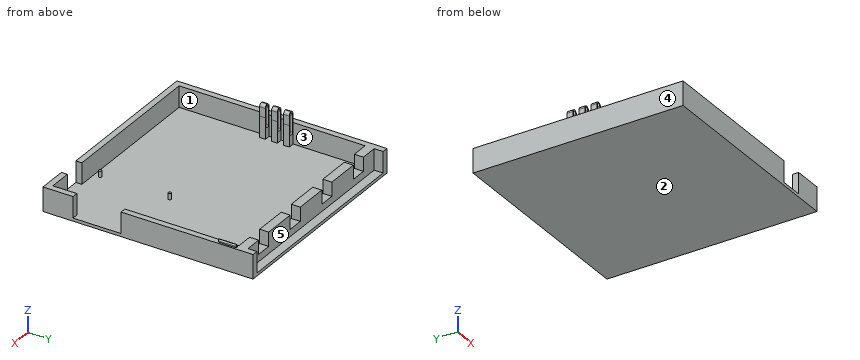
from build123d import *

# Parameters (mm, degrees)
F0_W           = 175
F0_H           = 175
F1_DEPTH       = 20
F2_W           = 165
F2_H           = 155
F3_DEPTH       = 17.5
F4_R           = 1.25
F5_DEPTH       = 5
F6_W           = 165
F6_H           = 7.5
F7_DEPTH       = 17.5
F8_W           = 13.2
F8_H           = 5.7
F9_DEPTH       = 8.5
F10_W          = 5
F10_H          = 5
F11_DEPTH      = 17.5
F11_DEPTH_BACK = 10
F11_TAPER_BACK = 1
F12_T1_DEPTH   = 16.9346144904
F12_T3_DEPTH   = 16.9346144904
F12_T5_DEPTH   = 16.9346144904
F14_DEPTH      = 25
F15_W          = 19
F15_H          = 17.6808023453
F15_W_2        = 32.2772479057
F15_H_2        = 40
F16_DEPTH      = 17.5
F17_W          = 13.2
F17_H          = 5.9
F18_DEPTH      = 8.5
F19_W          = 2
F19_H          = 15
F20_DEPTH      = 2
F21_R          = 0.99999
F22_R          = 0.5


# Not quite as in the source:
# - a fillet or chamfer that OpenCascade refuses, or shapes differently, is made with other operations: its cross-section is extruded or revolved along the edge and cut away or added
# - a fillet or chamfer is up to 0.001 mm smaller than in the source, because OpenCascade refuses the exact size


with BuildPart() as f1:
    # F0 (on Top) → F1 (new body)
    with BuildSketch(Plane.XY):
        Rectangle(F0_W, F0_H)
    extrude(amount=F1_DEPTH)

    # F2 (on face) → F3 (cut)
    with BuildSketch(Plane.XY.offset(20)):
        with Locations((0, -5)):
            Rectangle(F2_W, F2_H)
    extrude(amount=-F3_DEPTH, mode=Mode.SUBTRACT)

    # F4 (on face) → F5 (join)
    with BuildSketch(Plane.XY.offset(2.5)):
        with Locations((28.5, -77.5)):
            Circle(F4_R)
        with Locations((28.5, -19.5)):
            Circle(F4_R)
        with Locations((77.5, -77.5)):
            Circle(F4_R)
        with Locations((77.5, -19.5)):
            Circle(F4_R)
    extrude(amount=F5_DEPTH)

    # F6 (on face) → F7 (cut)
    with BuildSketch(Plane.XY.offset(20)):
        with Locations((0, 83.75)):
            Rectangle(F6_W, F6_H)
    extrude(amount=-F7_DEPTH, mode=Mode.SUBTRACT)

    # F8 (on face) → F9 (cut)
    with BuildSketch(Plane(origin=(0, 80, 0), x_dir=(-1, 0, 0), z_dir=(0, 1, 0))):
        with Locations((-61.875, 11.25)):
            Rectangle(F8_W, F8_H)
        with Locations((-20.625, 11.25)):
            Rectangle(F8_W, F8_H)
        with Locations((20.625, 11.25)):
            Rectangle(F8_W, F8_H)
        with Locations((61.875, 11.25)):
            Rectangle(F8_W, F8_H)
    extrude(amount=-F9_DEPTH, mode=Mode.SUBTRACT)

    # F10 (on face) → F11 (join, two sides)
    with BuildSketch(Plane.XY.offset(20)) as f11_sk:
        with Locations((-80, 0)):
            Rectangle(F10_W, F10_H)
        with Locations((-80, 10)):
            Rectangle(F10_W, F10_H)
        with Locations((-80, -10)):
            Rectangle(F10_W, F10_H)
    extrude(amount=-F11_DEPTH)
    extrude(f11_sk.sketch, amount=F11_DEPTH_BACK, taper=F11_TAPER_BACK)

    # F12: fillet of radius 2.5 on 6 edges, made by hand

    # F12_s2 → F12_t1 (cut)
    with BuildSketch(Plane.XZ.offset(-18.4673072452)):
        with BuildLine():
            ThreePointArc((-82.3683254308, 27.5436310161), (-81.6209793537, 29.2831261229), (-79.8687061929, 30))
            Line((-79.8687061929, 30), (-82.3254493507, 30))
            Line((-82.3254493507, 30), (-82.3683254308, 27.5436310161))
        make_face()
        with BuildLine():
            ThreePointArc((-80.1312938071, 30), (-78.3790206463, 29.2831261229), (-77.6316745692, 27.5436310161))
            Line((-77.6316745692, 27.5436310161), (-77.6745506493, 30))
            Line((-77.6745506493, 30), (-80.1312938071, 30))
        make_face()
    extrude(amount=F12_T1_DEPTH, mode=Mode.SUBTRACT)

    # F12_s4 → F12_t3 (cut)
    with BuildSketch(Plane.XZ.offset(-8.4673072452)):
        with BuildLine():
            ThreePointArc((-82.3683254308, 27.5436310161), (-81.6209793537, 29.2831261229), (-79.8687061929, 30))
            Line((-79.8687061929, 30), (-82.3254493507, 30))
            Line((-82.3254493507, 30), (-82.3683254308, 27.5436310161))
        make_face()
        with BuildLine():
            ThreePointArc((-80.1312938071, 30), (-78.3790206463, 29.2831261229), (-77.6316745692, 27.5436310161))
            Line((-77.6316745692, 27.5436310161), (-77.6745506493, 30))
            Line((-77.6745506493, 30), (-80.1312938071, 30))
        make_face()
    extrude(amount=F12_T3_DEPTH, mode=Mode.SUBTRACT)

    # F12_s6 → F12_t5 (cut)
    with BuildSketch(Plane.XZ.offset(1.5326927548)):
        with BuildLine():
            ThreePointArc((-82.3683254308, 27.5436310161), (-81.6209793537, 29.2831261229), (-79.8687061929, 30))
            Line((-79.8687061929, 30), (-82.3254493507, 30))
            Line((-82.3254493507, 30), (-82.3683254308, 27.5436310161))
        make_face()
        with BuildLine():
            ThreePointArc((-80.1312938071, 30), (-78.3790206463, 29.2831261229), (-77.6316745692, 27.5436310161))
            Line((-77.6316745692, 27.5436310161), (-77.6745506493, 30))
            Line((-77.6745506493, 30), (-80.1312938071, 30))
        make_face()
    extrude(amount=F12_T5_DEPTH, mode=Mode.SUBTRACT)

    # F13 (on face) → F14 (cut)
    with BuildSketch(Plane(origin=(0, 12.5, 0), x_dir=(-1, 0, 0), z_dir=(0, 1, 0))):
        with BuildLine():
            Line((81.5, 12.5), (81.5, 27.5))
            ThreePointArc((81.5, 27.5), (80, 29), (78.5, 27.5))
            Line((78.5, 27.5), (78.5, 12.5))
            ThreePointArc((78.5, 12.5), (80, 11), (81.5, 12.5))
        make_face()
    extrude(amount=-F14_DEPTH, mode=Mode.SUBTRACT)

    # F15 (on face) → F16 (cut)
    with BuildSketch(Plane.XY.offset(20)):
        with Locations((54, -82.5)):
            Rectangle(F15_W, F15_H)
        with Locations((82.5, -42.5)):
            Rectangle(F15_W_2, F15_H_2)
    extrude(amount=-F16_DEPTH, mode=Mode.SUBTRACT)

    # F17 (on face) → F18 (cut)
    with BuildSketch(Plane(origin=(0, 80, 0), x_dir=(-1, 0, 0), z_dir=(0, 1, 0))):
        with Locations((-61.875, 17.05)):
            Rectangle(F17_W, F17_H)
        with Locations((-20.625, 17.05)):
            Rectangle(F17_W, F17_H)
        with Locations((20.625, 17.05)):
            Rectangle(F17_W, F17_H)
        with Locations((61.875, 17.05)):
            Rectangle(F17_W, F17_H)
    extrude(amount=-F18_DEPTH, mode=Mode.SUBTRACT)

    # F19 (on face) → F20 (join)
    with BuildSketch(Plane.XY.offset(20)):
        with Locations((85, 65)):
            Rectangle(F19_W, F19_H)
    extrude(amount=F20_DEPTH)

    # F21 (radius 1 in the source; OpenCascade refuses exactly that, so slightly less here)
    f21_edges = [f1.edges().sort_by_distance(p)[0] for p in [
        (84, 65, 22),
        (86, 65, 22),
    ]]
    fillet(f21_edges, radius=F21_R)

    # F22
    f22_edges = [f1.edges().sort_by_distance(p)[0] for p in [
        (85.70711, 57.5, 21.70711),
        (85.70711, 72.5, 21.70711),
        (86, 57.5, 20.500005),
        (86, 72.5, 20.500005),
        (84, 57.5, 20.500005),
        (84.29289, 57.5, 21.70711),
        (85, 57.5, 22),
        (85, 72.5, 22),
        (84, 72.5, 20.500005),
        (84.29289, 72.5, 21.70711),
    ]]
    fillet(f22_edges, radius=F22_R)


solid = f1.part
CAD build for the part. Positions are in the model's coordinates, mm. Face numbers are marked on the shaded views. A direction names the side the tool comes from. Round coordinates to 2 decimals unless told otherwise and drop trailing zeros. Loops run counter-clockwise (first coordinate to the right, second up) from the corner with the lowest first, then second, coordinate; pieces in that order, holes last.
(1) Cut at C-C (z = 17.5). State how many separate pieces and enclosed holes the cut face has, plus the area to 3 significant figures.
(2) Cut at A-A (y = -37.5). Give the cut face in (x, z).
(3) Wall check: line 1 along X through (y, z) = (-66.5, 9.5); line 2 along Y through (x, z) = (-44, 12); line 3 along X through (y, z) = (10, 11.5). Give the ranges that are in metal, low to high.
(4) Cut at B-B (x = -1.5). Give the cut face in (y, z).
(5) Cut at D-D (y = 51.5). Give the cut face in (x, z).
(6) Which spindle directions (+Z, -Z, +X, -X, +Y, -Y) get a long thin tool onto all of the face, cutting with end or side? Do the marked faces 1 and 2. Say none if no direction does.
(7) Two-plate mould, pull along Y, no slides. Class the marked faces 3, 4 and 5: +Y half, -Y half, draft (parallel to the pull), parting line (faces both ways), or undercut.
(8) Drop flat-ended pins along their axis: pin 1 (5 mm diameter, centred on x = 30.5, z = 13.5, fed in from +Y); pin 2 (2 mm diameter, centred on x = 28.5, y = -78, fed in from +Z); pin 3 (5.5 mm diameter, centred on y = 0, z = 23.5, fed in from +X). Give the stop position or say it passes through.
Findings below:
1. separate pieces: 9
1. enclosed holes: 0
1. area: 3,150 mm2
2. outline: (-87.5, 0) - (87.5, 0) - (87.5, 2.5) - (-82.5, 2.5) - (-82.5, 20) - (-87.5, 20) - close
3. line 1: x = -87.5 to -82.5, 82.5 to 87.5
3. line 2: y = -87.5 to -82.5, 72.5 to 80
3. line 3: x = -87.5 to -81.12, -78.88 to -77.5, 82.5 to 87.5
4. outline: (-87.5, 0) - (87.5, 0) - (87.5, 2.5) - (80, 2.5) - (80, 20) - (72.5, 20) - (72.5, 2.5) - (-82.5, 2.5) - (-82.5, 20) - (-87.5, 20) - close
5. outline: (-87.5, 0) - (87.5, 0) - (87.5, 20) - (82.5, 20) - (82.5, 2.5) - (-82.5, 2.5) - (-82.5, 20) - (-87.5, 20) - close
6. face 1: +Z
6. face 2: -Z, +X, -X, +Y, -Y
7. face 3: undercut
7. face 4: draft
7. face 5: +Y half
8. pin 1: stops at y = 80
8. pin 2: stops at z = 7.5
8. pin 3: stops at x = -77.51
